Source: CAD feature listing. Evaluate the final solid. Frame: model axes, mm. A direction names the side the tool comes from. Give positions to 0.01 mm unless a question says otherwise; leave off trailing zeros. Write each loop counter-clockwise with the first axis right and the second up, starting at its lowest first coordinate (ties: lowest second). Pieces come first, ordered by that corner, then holes. Notation, with made-up numbers: (1.5, -5) -> (34.5, -5) arc R9 ccw to (34.5, 12) -> close; hole circle Ø11 at (-32.5, 89). An arc over 180 degrees is marked (long way). Answer as a JSON object with one key per item and string values. Group by question number.
Item 1: Section query C-C on x = 49. Return the cut outline in (y, z).
Item 2: Ray query, probe 1 along Y at (x, z) = (61.5, -7.5); probe 2 along X at (y, z) = (100.5, -11.5); probe 3 along Z at (x, y) = (-26, -200.5). Return the intervals inside material, ascending. Write a range as from..to.
Item 3: Section query A-A on z = -7. Return the cut outline in (x, y).
Item 4: First-contact query: pin 1 Ø0.8 at (x, z) = (-276.5, -0.5) entering from -Y; pin 2 Ø1.6 at (x, z) = (276.5, -0.5) entering from -Y; pin 3 Ø1.2 at (x, z) = (276, -0.5) entering from +Y. Flat tips, straight axial feed; report the tip coordinate or a pass-through.
Item 5: Section query B-B on y = 152.5. Return the cut outline in (x, z), plus the area to 3 significant figures.
Item 6: Access query for faces 1 (the face through (276, 4, -9)), 2 (the face through (4, -276.5, -9)), 3 (the face through (4, -278, -8)). Directions: +Z, -Z, +X, -X, +Y, -Y. A direction counts if a zero-diameter tool reaches every point of the face in a straight line with its end or side. Return the directions, or none.
Item 7: Pull-direction query (X, two-part tool) for faces 4 (the face through (-4, 4, -1.5)), 5 (the face through (-277.5, -4, -8)), 6 (the face through (-4, 276.5, -9)); classes: pulls with the +X half, pulls with the -X half, needs draft (parallel to the pull), parting line crosses it, or undercut.
from build123d import *

# Parameters (mm, degrees)
SKETCH_2_W                         = 555
SKETCH_2_H                         = 556
SM_BASE_FLANGE_1_DEPTH             = 1.5
SM_EDGE_FLANGE_2_STRIP_W           = 7
SM_EDGE_FLANGE_2_STRIP_H           = 1.5
SM_EDGE_FLANGE_2_STRIP_CUT_DEPTH   = 555
SM_EDGE_FLANGE_2_STRIP_2_W         = 7
SM_EDGE_FLANGE_2_STRIP_2_H         = 1.5
SM_EDGE_FLANGE_2_STRIP_CUT_2_DEPTH = 555
SM_EDGE_FLANGE_2_DEPTH             = 555
SM_EDGE_FLANGE_2_BEND_DEPTH        = 555
SM_EDGE_FLANGE_3_STRIP_W           = 7
SM_EDGE_FLANGE_3_STRIP_H           = 1.5
SM_EDGE_FLANGE_3_STRIP_CUT_DEPTH   = 552
SM_EDGE_FLANGE_3_STRIP_2_W         = 7
SM_EDGE_FLANGE_3_STRIP_2_H         = 1.5
SM_EDGE_FLANGE_3_STRIP_CUT_2_DEPTH = 552
SM_EDGE_FLANGE_3_DEPTH             = 552
SM_EDGE_FLANGE_3_BEND_DEPTH        = 552


# Sheet-metal steps are written as plain solids
with BuildPart() as part:
    # Sketch 2 → 基体-法兰1 (new body)
    with BuildSketch(Plane.XY):
        Rectangle(SKETCH_2_W, SKETCH_2_H)
    extrude(amount=-SM_BASE_FLANGE_1_DEPTH)

    # 边线-法兰2 strip (across the edge) → 边线-法兰2 strip cut (cut)
    with BuildSketch(Plane(origin=(-277.5, 278, -1.5), x_dir=(0, -1, 0), z_dir=(1, 0, 0))):
        with Locations((-1.5, -0.75)):
            Rectangle(SM_EDGE_FLANGE_2_STRIP_W, SM_EDGE_FLANGE_2_STRIP_H)
    extrude(amount=SM_EDGE_FLANGE_2_STRIP_CUT_DEPTH, mode=Mode.SUBTRACT)

    # 边线-法兰2 strip 2 (across the edge) → 边线-法兰2 strip cut 2 (cut)
    with BuildSketch(Plane(origin=(277.5, -278, -1.5), x_dir=(0, 1, 0), z_dir=(-1, 0, 0))):
        with Locations((-1.5, -0.75)):
            Rectangle(SM_EDGE_FLANGE_2_STRIP_2_W, SM_EDGE_FLANGE_2_STRIP_2_H)
    extrude(amount=SM_EDGE_FLANGE_2_STRIP_CUT_2_DEPTH, mode=Mode.SUBTRACT)

    # 边线-法兰2 section (across the edge) → 边线-法兰2 (add)
    with BuildSketch(Plane(origin=(-277.5, 278, -1.5), x_dir=(0, -1, 0), z_dir=(1, 0, 0))):
        with BuildLine():
            Line((0, 0.5), (0, 13.5))
            Line((0, 13.5), (1.5, 13.5))
            Line((1.5, 13.5), (1.5, 0.5))
            ThreePointArc((1.5, 0.5), (1.646446609, 0.146446609), (2, 0))
            Line((2, 0), (2, -1.5))
            ThreePointArc((2, -1.5), (0.585786438, -0.914213562), (0, 0.5))
        make_face()
    extrude(amount=SM_EDGE_FLANGE_2_DEPTH)

    # 边线-法兰2 section 2 (across the edge) → 边线-法兰2 bend (add)
    with BuildSketch(Plane(origin=(277.5, -278, -1.5), x_dir=(0, 1, 0), z_dir=(-1, 0, 0))):
        with BuildLine():
            Line((0, 0.5), (0, 13.5))
            Line((0, 13.5), (1.5, 13.5))
            Line((1.5, 13.5), (1.5, 0.5))
            ThreePointArc((1.5, 0.5), (1.646446609, 0.146446609), (2, 0))
            Line((2, 0), (2, -1.5))
            ThreePointArc((2, -1.5), (0.585786438, -0.914213562), (0, 0.5))
        make_face()
    extrude(amount=SM_EDGE_FLANGE_2_BEND_DEPTH)

    # 边线-法兰3 strip (across the edge) → 边线-法兰3 strip cut (cut)
    with BuildSketch(Plane(origin=(-277.5, -276, -1.5), x_dir=(1, 0, 0), z_dir=(0, 1, 0))):
        with Locations((-1.5, -0.75)):
            Rectangle(SM_EDGE_FLANGE_3_STRIP_W, SM_EDGE_FLANGE_3_STRIP_H)
    extrude(amount=SM_EDGE_FLANGE_3_STRIP_CUT_DEPTH, mode=Mode.SUBTRACT)

    # 边线-法兰3 strip 2 (across the edge) → 边线-法兰3 strip cut 2 (cut)
    with BuildSketch(Plane(origin=(277.5, 276, -1.5), x_dir=(-1, 0, 0), z_dir=(0, -1, 0))):
        with Locations((-1.5, -0.75)):
            Rectangle(SM_EDGE_FLANGE_3_STRIP_2_W, SM_EDGE_FLANGE_3_STRIP_2_H)
    extrude(amount=SM_EDGE_FLANGE_3_STRIP_CUT_2_DEPTH, mode=Mode.SUBTRACT)

    # 边线-法兰3 section (across the edge) → 边线-法兰3 (add)
    with BuildSketch(Plane(origin=(-277.5, -276, -1.5), x_dir=(1, 0, 0), z_dir=(0, 1, 0))):
        with BuildLine():
            Line((0, 0.5), (0, 13.5))
            Line((0, 13.5), (1.5, 13.5))
            Line((1.5, 13.5), (1.5, 0.5))
            ThreePointArc((1.5, 0.5), (1.646446609, 0.146446609), (2, 0))
            Line((2, 0), (2, -1.5))
            ThreePointArc((2, -1.5), (0.585786438, -0.914213562), (0, 0.5))
        make_face()
    extrude(amount=SM_EDGE_FLANGE_3_DEPTH)

    # 边线-法兰3 section 2 (across the edge) → 边线-法兰3 bend (add)
    with BuildSketch(Plane(origin=(277.5, 276, -1.5), x_dir=(-1, 0, 0), z_dir=(0, -1, 0))):
        with BuildLine():
            Line((0, 0.5), (0, 13.5))
            Line((0, 13.5), (1.5, 13.5))
            Line((1.5, 13.5), (1.5, 0.5))
            ThreePointArc((1.5, 0.5), (1.646446609, 0.146446609), (2, 0))
            Line((2, 0), (2, -1.5))
            ThreePointArc((2, -1.5), (0.585786438, -0.914213562), (0, 0.5))
        make_face()
    extrude(amount=SM_EDGE_FLANGE_3_BEND_DEPTH)


solid = part.part
Worked answers:
{
 "1": {"outline": "(-278, -15) -> (-276.5, -15) -> (-276.5, -2) arc R0.5 cw to (-276, -1.5) -> (276, -1.5) arc R0.5 cw to (276.5, -2) -> (276.5, -15) -> (278, -15) -> (278, -2) arc R2 ccw to (276, 0) -> (-276, 0) arc R2 ccw to (-278, -2) -> close"},
 "2": {"probe 1": "-278..-276.5, 276.5..278", "probe 2": "-277.5..-276, 276..277.5", "probe 3": "-1.5..0"},
 "3": {"outline": "(-277.5, -278) -> (277.5, -278) -> (277.5, -276.5) -> (-277.5, -276.5) -> close; (-277.5, -276) -> (-276, -276) -> (-276, 276) -> (-277.5, 276) -> close; (-277.5, 276.5) -> (277.5, 276.5) -> (277.5, 278) -> (-277.5, 278) -> close; (276, -276) -> (277.5, -276) -> (277.5, 276) -> (276, 276) -> close"},
 "4": {"pin 1": "y = -277.67", "pin 2": "y = -277.87", "pin 3": "y = 277.79"},
 "5": {"outline": "(-277.5, -15) -> (-276, -15) -> (-276, -2) arc R0.5 cw to (-275.5, -1.5) -> (275.5, -1.5) arc R0.5 cw to (276, -2) -> (276, -15) -> (277.5, -15) -> (277.5, -2) arc R2 ccw to (275.5, 0) -> (-275.5, 0) arc R2 ccw to (-277.5, -2) -> close", "area": "871 mm^2"},
 "6": {"face 1": "-Z", "face 2": "-Z, +X, -X", "face 3": "+Z, -Z, +X, -X, -Y"},
 "7": {"face 4": "undercut", "face 5": "pulls with the -X half", "face 6": "needs draft"}
}
